Geometry check sheet. Reference: the model listing, model coordinates, mm. A direction names the side the tool comes from. Round coordinates to 2 decimals unless told otherwise and drop trailing zeros. Write each loop counter-clockwise with the first axis right and the second up, starting at its lowest first coordinate (ties: lowest second). Pieces come first, ordered by that corner, then holes. Notation, with made-up numbers: (68.5, 36) -> (124.5, 36) arc R24 ccw to (124.5, 67) -> close; hole circle Ø9 at (10.25, 44.25). An arc over 180 degrees is marked (long way). Put each result on its own line as item: value. Start each with the question number.
from build123d import *

# Parameters (mm, degrees)
SKETCH1_R           = 2.15
BOSS_EXTRUDE1_DEPTH = 15


with BuildPart() as part:
    # Sketch1 → Boss-Extrude1 (new body)
    with BuildSketch(Plane(origin=(0, 0, 0), x_dir=(1, 0, 0), z_dir=(0, 1, 0))):
        Polygon((0, 0), (60, 0), (60, 20), (20, 20), (20, 60), (0, 60), align=None)
        with Locations(Location((50, 10, 0), (0, 0, 270))):
            Circle(SKETCH1_R, mode=Mode.SUBTRACT)
        with Locations(Location((30, 10, 0), (0, 0, 270))):
            Circle(SKETCH1_R, mode=Mode.SUBTRACT)
        with Locations(Location((10, 50, 0), (0, 0, 270))):
            Circle(SKETCH1_R, mode=Mode.SUBTRACT)
        with Locations(Location((10, 30, 0), (0, 0, 270))):
            Circle(SKETCH1_R, mode=Mode.SUBTRACT)
    extrude(amount=BOSS_EXTRUDE1_DEPTH)


solid = part.part
(1) Sectioned sample at B-B (z = -50). Record the cut outline in (x, y).
(2) Sectioned sample at A-A (x = 50). Record the cut outline in (y, z), and give its area (4 significant figures).
(3) Mould release check, pull along X, two halves, no side actions. Record for faces 3 (the flat face through (0, 7, -30)), 4 (the cylindrical face through (51.81, 7.4, -8.84)), 5 (the cylindrical face through (10.65, 7.4, -47.95)), 6 (the flat face through (40, 7, -20)): +X half, -X half, draft (parallel to the pull), parting line (faces both ways), or undercut.
(4) Set-up check for faces 1 (the flat face through (20, 7, -40)), 2 (the cylindrical face through (31.81, 7.4, -8.84)): record each of +Z, -Z, +X, -X, +Y, -Y from which the full face is reachable in a straight line by a thin tool's end or side.
(5) Go/stop test with flat-tipped pins: pin 1 Ø1.5 at (x, z) = (8, -49) entering from -Y; pin 2 Ø1.5 at (x, y) = (30, 5) entering from -Z; pin 3 Ø4.5 at (y, z) = (6.5, -33) entering from +X. Record where each tip stops, or that it passes through.
(6) Sectioned sample at C-C (z = -10). Record the cut outline in (x, y).
(7) Material ranges on L1, parallel to X at y = 5, z = -10; L2, parallel to X at y = 9, z = -30; L3, parallel to X at y = 10.75, z = -22, recorded low to high. Write a range as from..to.
(8) Sectioned sample at D-D (x = 10). Record the cut outline in (y, z).
Found:
1. outline: (0, 0) -> (7.85, 0) -> (7.85, 15) -> (0, 15) -> close; (12.15, 0) -> (20, 0) -> (20, 15) -> (12.15, 15) -> close
2. outline: (0, -20) -> (15, -20) -> (15, -12.15) -> (0, -12.15) -> close; (0, -7.85) -> (15, -7.85) -> (15, 0) -> (0, 0) -> close
2. area: 235.5 mm2
3. face 3: -X half
3. face 4: undercut
3. face 5: undercut
3. face 6: draft
4. face 1: -Z, +X, +Y, -Y
4. face 2: +Y, -Y
5. pin 1: y = 0
5. pin 2: z = -20
5. pin 3: x = 20
6. outline: (0, 0) -> (27.85, 0) -> (27.85, 15) -> (0, 15) -> close; (32.15, 0) -> (47.85, 0) -> (47.85, 15) -> (32.15, 15) -> close; (52.15, 0) -> (60, 0) -> (60, 15) -> (52.15, 15) -> close
7. L1: 0..27.85, 32.15..47.85, 52.15..60
7. L2: 0..7.85, 12.15..20
7. L3: 0..20
8. outline: (0, -60) -> (15, -60) -> (15, -52.15) -> (0, -52.15) -> close; (0, -47.85) -> (15, -47.85) -> (15, -32.15) -> (0, -32.15) -> close; (0, -27.85) -> (15, -27.85) -> (15, 0) -> (0, 0) -> close
